Input: part model. Units: mm. Frame: model coordinates. A direction names the side the tool comes from. Give positions to 0.01 mm unless a question says otherwise; leave off trailing zeros. Loops run counter-clockwise (first coordinate to the right, second up) from the corner with the lowest first, then second, coordinate; pieces in that order, holes last. Notation, with made-up numbers: (-24, 68) -> (21, 68) arc R31 ccw to (21, 104) -> close; hole circle Ø3 at (32.5, -38). An arc over 180 degrees is marked (long way). Answer in a Markdown table with one row per item. Add a question column.
Autodesk Inventor part; units mm, degrees
ref_plane "Work Plane1" through (0, -25.4, 0) normal (0, 1, 0) x (1, 0, 0)
ref_plane "YZ Plane" through (0, 0, 0) normal (1, 0, 0) x (0, 1, 0)
ref_plane "XZ Plane" through (0, 0, 0) normal (0, 1, 0) x (-1, 0, 0)
sketch "Sketch1" plane through (0, 0, 0) normal (0, 1, 0) x (-1, 0, 0)
  line L0 (-462.2267, 0) -> (462.2267, 0)
  line L1 (0, -462.2267) -> (0, 462.2267)
  line L2 (-330.1619, 330.1619) -> (330.1619, 330.1619)
  line L3 (330.1619, 330.1619) -> (330.1619, -330.1619)
  line L4 (330.1619, -330.1619) -> (-330.1619, -330.1619)
  line L5 (-330.1619, -330.1619) -> (-330.1619, 330.1619)
  line L6 (462.2267, 0) -> (-462.2267, 0)
  line L7 (0, -462.2267) -> (0, 462.2267)
  line L8 (314.2869, -314.2869) -> (-314.2869, -314.2869)
  line L9 (-314.2869, -314.2869) -> (-314.2869, 314.2869)
  line L10 (-314.2869, 314.2869) -> (314.2869, 314.2869)
  line L11 (314.2869, 314.2869) -> (314.2869, -314.2869)
  point P0 (0, 0)
  dimension "d0" = 660.3238
  dimension "d2" = 660.3238
  dimension "d123" = 15.875
  dimension "d124" = 15.875
extrude "Extrusion1" add sketch "Sketch1" against normal blind 1.5875 contours L5 L2 L1 L10 L9 L0 | L0 L9 L8 L1 L4 L5 | L1 L8 L11 L0 L3 L4 | L2 L3 L0 L11 L10 L1
sketch "Sketch2" plane through (0, -1.5875, 0) normal (0, -1, 0) x (1, 0, 0)
  line L0 (330.1619, 330.1619) -> (-330.1619, 330.1619)
  line L1 (-330.1619, 330.1619) -> (-330.1619, -330.1619)
  line L2 (-330.1619, -330.1619) -> (330.1619, -330.1619)
  line L3 (330.1619, -330.1619) -> (330.1619, 330.1619)
  line L4 (-314.2869, -314.2869) -> (-314.2869, 314.2869)
  line L5 (-314.2869, 314.2869) -> (314.2869, 314.2869)
  line L6 (314.2869, 314.2869) -> (314.2869, -314.2869)
  line L7 (314.2869, -314.2869) -> (-314.2869, -314.2869)
  line L8 (330.1619, 330.1619) -> (-330.1619, 330.1619)
  line L9 (-330.1619, 330.1619) -> (-330.1619, -330.1619)
  line L10 (-330.1619, -330.1619) -> (330.1619, -330.1619)
  line L11 (330.1619, -330.1619) -> (330.1619, 330.1619)
  line L12 (0, -462.2267) -> (0, 462.2267)
  line L13 (-462.2267, 0) -> (462.2267, 0)
  line L14 (-328.5744, 328.5744) -> (328.5744, 328.5744)
  line L15 (328.5744, 328.5744) -> (328.5744, -328.5744)
  line L16 (328.5744, -328.5744) -> (-328.5744, -328.5744)
  line L17 (-328.5744, -328.5744) -> (-328.5744, 328.5744)
  point P0 (0, 0)
  dimension "d7" = 1.5875
  dimension "d8" = 1.5875
extrude "Extrusion2" add sketch "Sketch2" along normal blind 136.525 contours L3 L13 L15 L14 L12 L0 | L12 L14 L17 L13 L1 L0 | L3 L2 L12 L16 L15 L13 | L13 L17 L16 L12 L2 L1
sketch "Sketch3" plane through (0, -138.1125, 0) normal (0, -1, 0) x (1, 0, 0)
  line L0 (-462.2267, 0) -> (462.2267, 0)
  line L1 (0, -462.2267) -> (0, 462.2267)
  line L2 (-330.1619, 330.1619) -> (330.1619, 330.1619)
  line L3 (330.1619, 330.1619) -> (330.1619, -330.1619)
  line L4 (330.1619, -330.1619) -> (-330.1619, -330.1619)
  line L5 (-330.1619, -330.1619) -> (-330.1619, 330.1619)
  point P0 (0, 0)
extrude "Extrusion3" add sketch "Sketch3" along normal blind 1.5875
ref_plane "Work Plane1" through (0, -25.4, 0) normal (0, 1, 0) x (1, 0, 0)
sketch "Sketch4" plane through (0, -25.4, 0) normal (0, 1, 0) x (1, 0, 0)
  line L0 (328.5744, -328.5744) -> (328.5744, 328.5744)
  line L1 (328.5744, 328.5744) -> (-328.5744, 328.5744)
  line L2 (-328.5744, 328.5744) -> (-328.5744, -328.5744)
  line L3 (-328.5744, -328.5744) -> (328.5744, -328.5744)
  line L4 (-330.1619, -330.1619) -> (-330.1619, 330.1619)
  line L5 (-330.1619, 330.1619) -> (330.1619, 330.1619)
  line L6 (330.1619, 330.1619) -> (330.1619, -330.1619)
  line L7 (330.1619, -330.1619) -> (-330.1619, -330.1619)
  line L8 (-288.8869, 288.8869) -> (288.8869, 288.8869)
  line L9 (288.8869, 288.8869) -> (288.8869, -288.8869)
  line L10 (288.8869, -288.8869) -> (-288.8869, -288.8869)
  line L11 (-288.8869, -288.8869) -> (-288.8869, 288.8869)
  line L12 (462.2267, 0) -> (-462.2267, 0)
  line L13 (0, 462.2267) -> (0, -462.2267)
  point P0 (0, 0)
  dimension "d121" = 41.275
  dimension "d122" = 41.275
extrude "Extrusion4" add sketch "Sketch4" against normal blind 1.5875 contours L3 L13 L10 L9 L12 L0 | L12 L9 L8 L13 L1 L0 | L3 L2 L12 L11 L10 L13 | L13 L8 L11 L12 L2 L1
fillet "Fillet1" radius 3.175 12 edges at (0, 0, 330.1619) (0, -139.7, 330.1619) (330.1619, -69.85, 330.1619) (330.1619, -139.7, 0) (330.1619, 0, 0) (330.1619, -69.85, -330.1619) (0, 0, -330.1619) (-330.1619, 0, 0) (-330.1619, -69.85, 330.1619) (0, -139.7, -330.1619) (-330.1619, -69.85, -330.1619) (-330.1619, -139.7, 0)
sketch "Sketch11" plane through (0, -139.7, 0) normal (0, -1, 0) x (1, 0, 0)
  line L0 (326.9869, -326.9869) -> (-326.9869, -326.9869)
  line L1 (0, 462.2267) -> (0, -462.2267)
  circle A0 centre (0, -250.7869) radius 16.7005
  point P0 (0, 0)
  dimension "d130" = 33.401
  dimension "d131" = 76.2
  dimension "d74" = 57.15
  dimension "d75" = 33.401
extrude "Extrusion12" cut sketch "Sketch11" against normal up to next
sketch "Sketch6" plane through (-328.5744, -138.1125, -328.5744) normal (0, 0, 1) x (1, 0, 0)
  circle A0 centre (298.4119, 42.8625) radius 15.875
  circle A1 centre (298.4119, 42.8625) radius 15.875
  circle A2 centre (298.4119, 42.8625) radius 12.7
  point P0 (328.5744, 138.1125)
  dimension "d83" = 25.4
sketch "Sketch7" plane through (330.1619, -136.525, 326.9869) normal (1, 0, 0) x (0, 0, -1)
  line L0 (653.9738, 136.525) -> (0, 136.525)
  line L1 (326.9869, -34.925) -> (326.9869, 187.325)
  circle A0 centre (55.5752, 152.4) radius 3.175
  line L2 (-1.5875, 134.9375) -> (-1.5875, 111.125)
  line L3 (-3.175, 133.35) -> (-3.175, 0)
  circle A1 centre (598.3986, 152.4) radius 3.175
  point P0 (326.9869, 136.525)
  dimension "d91" = 6.35
  dimension "d95" = 58.7502
  dimension "d96" = 15.875
properties part number "Propane Burner Base" material "Steel"
1) Pin query (flat end, axial travel): pin 1 (0.8 mm diameter, centred on y = -0.5, z = -81, fed in from +X); pin 2 (1.3 mm diameter, centred on x = -42.5, y = -1, fed in from +Z); pin 3 (1.3 mm diameter, centred on x = -89.5, y = -0.5, fed in from -Z). Return the tip coordinate at first contact, or that it passes through.
2) Reachability of faces 5 (the face through (328.574, -82, 5)), 6 (the face through (-2.174, -138.917, -234.229)) from +Z, -Z, +X, -X, +Y, -Y: full face, straight path, thin tool, end or side. Return the list, or none.
3) Pull-direction query (Y, two-part tool) for faces 1 (the face through (147, 0, 316)), 2 (the face through (-5, -139.7, 5)), 3 (the face through (-5, -69, -330.162)), 4 (the face through (-5, -13, 328.574)); classes: +Y half, -Y half, draft (parallel to the pull), parting line (faces both ways), or undercut.
4) Material intervals for line 1 along Z through (x, y) = (-75, -106); line 2 along Y through (x, z) = (302.5, 201), sorted ascending.
5) Section A-A on y = -80. Output: boundary loops of the cut face in (x, z) (3 decimals), and give its area (3 significant figures).
Working result:
| question | item | result |
|---|---|---|
| 1 | pin 1 | stops at x = 329.2 |
| 1 | pin 2 | stops at z = 329.77 |
| 1 | pin 3 | stops at z = -329.43 |
| 2 | face 5 | none |
| 2 | face 6 | +Y, -Y |
| 3 | face 1 | +Y half |
| 3 | face 2 | -Y half |
| 3 | face 3 | draft |
| 3 | face 4 | undercut |
| 4 | line 1 | z = -330.16 to -328.57, 328.57 to 330.16 |
| 4 | line 2 | y = -139.7 to -138.11, -26.99 to -25.4 |
| 5 | outline | (-330.162, -326.987) arc R3.175 ccw to (-326.987, -330.162) -> (326.987, -330.162) arc R3.175 ccw to (330.162, -326.987) -> (330.162, 326.987) arc R3.175 ccw to (326.987, 330.162) -> (-326.987, 330.162) arc R3.175 ccw to (-330.162, 326.987) -> close; hole (-328.574, -328.574) -> (328.574, -328.574) -> (328.574, 328.574) -> (-328.574, 328.574) -> close |
| 5 | area | 4,170 mm2 |
